```python
from build123d import *

# Parameters (mm, degrees)
SKETCH2_R          = 9.525
SKETCH6_R          = 6.35
CUT_EXTRUDE1_DEPTH = 139.7


with BuildPart() as part:
    # Sweep1: sweep along a path in Sketch1
    with BuildLine(Plane.XY) as sweep1_path:
        Line((0, 0), (0, 101.6))
        ThreePointArc((0, 101.6), (7.439487758, 119.560512242), (25.4, 127))
        Line((25.4, 127), (63.845922056, 127))
        ThreePointArc((63.845922056, 127), (74.955603314, 124.441518827), (83.827181396, 117.281494672))
        Line((83.827181396, 117.281494672), (155.936708861, 25.4))
        ThreePointArc((155.936708861, 25.4), (162.997624279, 19.70131545), (171.839852681, 17.665012665))
        Line((171.839852681, 17.665012665), (298.839852681, 17.665012665))
    # Sketch2 → Sweep1 (sweep)
    with BuildSketch(Plane(origin=(0, 0, 0), x_dir=(1, 0, 0), z_dir=(0, 1, 0))):
        Circle(SKETCH2_R)
    sweep(path=sweep1_path.line)

    # Sketch6 → Cut-Extrude1 (cut)
    with BuildSketch(Plane.XZ):
        with Locations(Location((0, 0, 0), (0, 0, 270))):
            Circle(SKETCH6_R)
    extrude(amount=-CUT_EXTRUDE1_DEPTH, mode=Mode.SUBTRACT)


solid = part.part
```
Geometry check sheet. Reference: the model listing, model coordinates, mm. A direction names the side the tool comes from. Coordinates: 2 decimals unless noted, no trailing zeros. Order: outer loops, then holes, each group sorted by start corner. A loop starts at its lowest first (then second) coordinate and runs counter-clockwise, first axis right, second up. Notation, with made-up numbers: M -26.75,37.5 L 10.25,37.5 A25 cw 10.25,76.5 Z; hole C 71.5,25 d4. An arc over 180 degrees is marked long. Answer as a JSON object with one key per item and string values.
Q1. Depth check by flat-ended pin: pin 1 Ø5 at (x, y) = (160.5, 13.5) entering from -Z; pin 2 Ø1 at (y, z) = (55, -4.5) entering from +X; pin 3 Ø2 at (x, z) = (28.5, 6) entering from +Y; pin 4 Ø8 at (y, z) = (94, -4) entering from -X (3 decimals). Enter the tip coordinate at first touch or a pass-through.
Results are:
{"pin 1": "stops at z = -8.56", "pin 2": "stops at x = 143.89", "pin 3": "stops at y = 135.11", "pin 4": "stops at x = -9.525"}
Q2. Tool access check on faces 1 (the cylindrical face through (236.23, 8.58, -2.86)), 2 (the cylindrical face through (44.892, 136.516, -0.419)), 3 (the flat face through (-6.2, 0, 2)). Record the directions out of +Z, -Z, +X, -X, +Y, -Y that give a thin tool (end or side, any length) a straight path to the whole face; none if there is none.
Results are:
{"face 1": "+X", "face 2": "none", "face 3": "+Z, -Z, +X, -X, -Y"}
Q3. Cross-section at A-A on z = 0. Record the cut outline in (x, y) (3 decimals).
Results are:
{"outline": "M -9.525,0 L -6.35,0 L -6.35,116.15 A34.925 ccw -9.525,101.6 Z; M 6.35,0 L 9.525,0 L 9.525,101.6 A15.875 cw 25.4,117.475 L 63.846,117.475 A15.875 cw 76.334,111.401 L 148.444,19.519 A29.741 ccw 171.84,8.14 L 298.84,8.14 L 298.84,27.19 L 171.84,27.19 A10.691 cw 163.43,31.281 L 91.32,123.162 A34.925 ccw 63.846,136.525 L 25.4,136.525 A34.925 ccw 6.35,130.872 Z"}
Q4. Cross-section at C-C on x = 182.5. Record the cut outline in (y, z) (3 decimals).
Results are:
{"outline": "C 17.665,0 d19.05"}
Q5. Release check for a two-part mould opening along Z. For faces 4 (the cylindrical face through (6.3, 64.5, 0.8)), 5 (the flat face through (298.84, 18, 0)), 6 (the cylindrical face through (-7.559, 51.511, 5.796)) record: released by +Z, released by -Z, zero draft, split by the parting line, or undercut.
Results are:
{"face 4": "undercut", "face 5": "zero draft", "face 6": "split by the parting line"}
Q6. Scan lines: line 1 (Z direction, x = 0, y = 73) (3 decimals); line 2 (X direction, y = 76, z = 0) (3 decimals); line 3 (Z direction, x = 117.5, y = 76). Record each from-to range of solid material in increasing order.
Results are:
{"line 1": "z = -9.525 to -6.35, 6.35 to 9.525", "line 2": "x = -9.525 to -6.35, 6.35 to 9.525, 104.117 to 128.333", "line 3": "z = -9.47 to 9.47"}
Q7. Cross-section at B-B on y = 23. Give the number of separate pieces and of enclosed holes in the cut face, and give its area (3 significant figures).
Results are:
{"separate pieces": "2", "enclosed holes": "1", "area": "2,590 mm²"}
